```python
from build123d import *

# Parameters (mm, degrees)
ESQUISSE1_W             = 60
ESQUISSE1_H             = 60
ESQUISSE1_R             = 1.65
BOSS_EXTRU_1_DEPTH      = 3
ESQUISSE2_W             = 8
ESQUISSE2_H             = 40
ENL_V_MAT_EXTRU_1_DEPTH = 3


with BuildPart() as part:
    # Esquisse1 → Boss.-Extru.1 (new body)
    with BuildSketch(Plane.XY):
        Rectangle(ESQUISSE1_W, ESQUISSE1_H)
        with Locations((-15, 25)):
            Circle(ESQUISSE1_R, mode=Mode.SUBTRACT)
        with Locations((5, 25)):
            Circle(ESQUISSE1_R, mode=Mode.SUBTRACT)
        with Locations((15, 25)):
            Circle(ESQUISSE1_R, mode=Mode.SUBTRACT)
        with Locations((-5, 25)):
            Circle(ESQUISSE1_R, mode=Mode.SUBTRACT)
        with Locations((-15, -27)):
            Circle(ESQUISSE1_R, mode=Mode.SUBTRACT)
        with Locations((-5, -27)):
            Circle(ESQUISSE1_R, mode=Mode.SUBTRACT)
        with Locations((5, -27)):
            Circle(ESQUISSE1_R, mode=Mode.SUBTRACT)
        with Locations((15, -27)):
            Circle(ESQUISSE1_R, mode=Mode.SUBTRACT)
    extrude(amount=-BOSS_EXTRU_1_DEPTH)

    # Esquisse2 → Enlèv. mat.-Extru.1 (cut)
    with BuildSketch(Plane.XY):
        with Locations((-16, 0)):
            Rectangle(ESQUISSE2_W, ESQUISSE2_H)
        Rectangle(ESQUISSE2_W, ESQUISSE2_H)
        with Locations((16, 0)):
            Rectangle(ESQUISSE2_W, ESQUISSE2_H)
    extrude(amount=-ENL_V_MAT_EXTRU_1_DEPTH, mode=Mode.SUBTRACT)


solid = part.part
```
The listing builds one solid part. Answer for the finished solid, in the listing's coordinates (mm). A direction names the side the tool comes from. Coordinates: 2 decimals unless noted, no trailing zeros. Write each loop counter-clockwise with the first axis right and the second up, starting at its lowest first coordinate (ties: lowest second). Pieces come first, ordered by that corner, then holes. Notation, with made-up numbers: (71, 0.5) - (99, 0.5) arc R18 ccw to (99, 18.5) - close; hole circle Ø9 at (-20.75, -25). An arc over 180 degrees is marked (long way). Return JSON: item names as keys, results as strings. Group by question number.
1. Which of the six approach directions +Z, -Z, +X, -X, +Y, -Y give full straight-line access (tool end or side, diameter ignored) to faces 5 (the flat face through (-7, 0, -3)), 6 (the flat face through (0, 20, -1))?
2. A cutting plane is placed at C-C, the plane x = -5. Determine the outline of the cut face in (y, z), plus the area to 3 significant figures.
3. Determine the mould class of faces 1 (the flat face through (-7, 0, 0)), 2 (the flat face through (0, 30, -1)), 3 (the cylindrical face through (-14.11, -25.61, -1.48)), 4 (the flat face through (20, 0, -1)) for opening direction Y: released by +Y, released by -Y, zero draft, split by the parting line, or undercut.
4. A cutting plane is placed at B-B, the plane z = -1.7. Give the number of separate pieces and of enclosed holes in the cut face, plus the area to 3 significant figures.
5. A cutting plane is placed at D-D, the plane y = 25. Determine the outline of the cut face in (x, z).
6. A cutting plane is placed at A-A, the plane y = -2.5. Determine the outline of the cut face in (x, z).
7. Straight lines are drawn through the part: L1, parallel to Y at x = -15, z = -1.05; L2, parallel to X at y = -19.5, z = -0.6; L3, parallel to Y at x = -5, z = -2.15. For each, find the intervals that lie inside material, in ascending order.
Ans:
{
 "1": {"face 5": "-Z, +X, -X, +Y, -Y", "face 6": "+Z, -Z"},
 "2": {"outline": "(-30, -3) - (-28.65, -3) - (-28.65, 0) - (-30, 0) - close; (-25.35, -3) - (23.35, -3) - (23.35, 0) - (-25.35, 0) - close; (26.65, -3) - (30, -3) - (30, 0) - (26.65, 0) - close", "area": "160 mm²"},
 "3": {"face 1": "zero draft", "face 2": "released by +Y", "face 3": "undercut", "face 4": "undercut"},
 "4": {"separate pieces": "1", "enclosed holes": "11", "area": "2,570 mm²"},
 "5": {"outline": "(-30, -3) - (-16.65, -3) - (-16.65, 0) - (-30, 0) - close; (-13.35, -3) - (-6.65, -3) - (-6.65, 0) - (-13.35, 0) - close; (-3.35, -3) - (3.35, -3) - (3.35, 0) - (-3.35, 0) - close; (6.65, -3) - (13.35, -3) - (13.35, 0) - (6.65, 0) - close; (16.65, -3) - (30, -3) - (30, 0) - (16.65, 0) - close"},
 "6": {"outline": "(-30, -3) - (-20, -3) - (-20, 0) - (-30, 0) - close; (-12, -3) - (-4, -3) - (-4, 0) - (-12, 0) - close; (4, -3) - (12, -3) - (12, 0) - (4, 0) - close; (20, -3) - (30, -3) - (30, 0) - (20, 0) - close"},
 "7": {"L1": "-30 to -28.65, -25.35 to -20, 20 to 23.35, 26.65 to 30", "L2": "-30 to -20, -12 to -4, 4 to 12, 20 to 30", "L3": "-30 to -28.65, -25.35 to 23.35, 26.65 to 30"}
}
